Check sheet for the modelled part. Datum: model origin and axes. Units: mm. A direction names the side the tool comes from. Round coordinates to 2 decimals unless told otherwise and drop trailing zeros. Write each loop counter-clockwise with the first axis right and the second up, starting at its lowest first coordinate (ties: lowest second). Pieces come first, ordered by that corner, then holes. Notation, with made-up numbers: M -1,-26.75 L 19,-26.75 A19 cw 19,0.25 Z; hole C -36,21.5 d3. An arc over 180 degrees is marked long. Put each result on its own line as item: value.
```python
from build123d import *

# Parameters (mm, degrees)
SKETCH_1_W          = 48.3
SKETCH_1_H          = 28.3
EXTRUDE_1_DEPTH     = 1.6
SKETCH_3_W          = 25.5
SKETCH_3_H          = 17.8
EXTRUDE_2_DEPTH     = 0.7
SKETCH_4_W          = 17.4
SKETCH_4_H          = 15.8
EXTRUDE_3_DEPTH     = 2.3
SKETCH_5_W          = 6.4
SKETCH_5_H          = 7.4
EXTRUDE_4_DEPTH     = 2.4
CHAMFER_1_SIZE      = 0.5
SKETCH_6_R          = 0.6
CUT_EXTRUDE_1_DEPTH = 34.530359378


with BuildPart() as part:
    # 草图1 → 凸台-拉伸1 (new body)
    with BuildSketch(Plane(origin=(0, 0, 0), x_dir=(1, 0, 0), z_dir=(0, 1, 0))):
        Rectangle(SKETCH_1_W, SKETCH_1_H)
    extrude(amount=EXTRUDE_1_DEPTH)

    # 草图3 → 凸台-拉伸2 (add)
    with BuildSketch(Plane(origin=(0, 1.6, 0), x_dir=(1, 0, 0), z_dir=(0, 1, 0))):
        with Locations((-17.5, 0)):
            Rectangle(SKETCH_3_W, SKETCH_3_H)
    extrude(amount=EXTRUDE_2_DEPTH)

    # 草图4 → 凸台-拉伸3 (add)
    with BuildSketch(Plane(origin=(0, 2.3, 0), x_dir=(1, 0, 0), z_dir=(0, 1, 0))):
        with Locations((-14.45, 0)):
            Rectangle(SKETCH_4_W, SKETCH_4_H)
    extrude(amount=EXTRUDE_3_DEPTH)

    # 草图5 → 凸台-拉伸4 (add)
    with BuildSketch(Plane(origin=(0, 1.6, 0), x_dir=(1, 0, 0), z_dir=(0, 1, 0))):
        with Locations((21.65, 0)):
            Rectangle(SKETCH_5_W, SKETCH_5_H)
    extrude(amount=EXTRUDE_4_DEPTH)

    # 倒角1
    chamfer_1_edges = [part.edges().sort_by_distance(p)[0] for p in [
        (21.65, 4, -3.7),
        (21.65, 4, 3.7),
    ]]
    chamfer(chamfer_1_edges, length=CHAMFER_1_SIZE)

    # 草图6 → 切除-拉伸1 (cut, through all)
    with BuildSketch(Plane(origin=(0, 1.6, 0), x_dir=(1, 0, 0), z_dir=(0, 1, 0))):
        with Locations(Location((22.95, 12.7, 0), (0, 0, 270))):
            Circle(SKETCH_6_R)
        with Locations(Location((20.41, 12.7, 0), (0, 0, 270))):
            Circle(SKETCH_6_R)
        with Locations(Location((17.87, 12.7, 0), (0, 0, 270))):
            Circle(SKETCH_6_R)
        with Locations(Location((15.33, 12.7, 0), (0, 0, 270))):
            Circle(SKETCH_6_R)
        with Locations(Location((12.79, 12.7, 0), (0, 0, 270))):
            Circle(SKETCH_6_R)
        with Locations(Location((10.25, 12.7, 0), (0, 0, 270))):
            Circle(SKETCH_6_R)
        with Locations(Location((7.71, 12.7, 0), (0, 0, 270))):
            Circle(SKETCH_6_R)
        with Locations(Location((5.17, 12.7, 0), (0, 0, 270))):
            Circle(SKETCH_6_R)
        with Locations(Location((2.63, 12.7, 0), (0, 0, 270))):
            Circle(SKETCH_6_R)
        with Locations(Location((0.09, 12.7, 0), (0, 0, 270))):
            Circle(SKETCH_6_R)
        with Locations(Location((-2.45, 12.7, 0), (0, 0, 270))):
            Circle(SKETCH_6_R)
        with Locations(Location((-4.99, 12.7, 0), (0, 0, 270))):
            Circle(SKETCH_6_R)
        with Locations(Location((-7.53, 12.7, 0), (0, 0, 270))):
            Circle(SKETCH_6_R)
        with Locations(Location((-10.07, 12.7, 0), (0, 0, 270))):
            Circle(SKETCH_6_R)
        with Locations(Location((-12.61, 12.7, 0), (0, 0, 270))):
            Circle(SKETCH_6_R)
        with Locations(Location((-15.15, 12.7, 0), (0, 0, 270))):
            Circle(SKETCH_6_R)
        with Locations(Location((-17.69, 12.7, 0), (0, 0, 270))):
            Circle(SKETCH_6_R)
        with Locations(Location((-20.23, 12.7, 0), (0, 0, 270))):
            Circle(SKETCH_6_R)
        with Locations(Location((-22.77, 12.7, 0), (0, 0, 270))):
            Circle(SKETCH_6_R)
        with Locations(Location((20.41, -12.7, 0), (0, 0, 270))):
            Circle(SKETCH_6_R)
        with Locations(Location((17.87, -12.7, 0), (0, 0, 270))):
            Circle(SKETCH_6_R)
        with Locations(Location((15.33, -12.7, 0), (0, 0, 270))):
            Circle(SKETCH_6_R)
        with Locations(Location((12.79, -12.7, 0), (0, 0, 270))):
            Circle(SKETCH_6_R)
        with Locations(Location((10.25, -12.7, 0), (0, 0, 270))):
            Circle(SKETCH_6_R)
        with Locations(Location((7.71, -12.7, 0), (0, 0, 270))):
            Circle(SKETCH_6_R)
        with Locations(Location((5.17, -12.7, 0), (0, 0, 270))):
            Circle(SKETCH_6_R)
        with Locations(Location((2.63, -12.7, 0), (0, 0, 270))):
            Circle(SKETCH_6_R)
        with Locations(Location((0.09, -12.7, 0), (0, 0, 270))):
            Circle(SKETCH_6_R)
        with Locations(Location((-2.45, -12.7, 0), (0, 0, 270))):
            Circle(SKETCH_6_R)
        with Locations(Location((-4.99, -12.7, 0), (0, 0, 270))):
            Circle(SKETCH_6_R)
        with Locations(Location((-7.53, -12.7, 0), (0, 0, 270))):
            Circle(SKETCH_6_R)
        with Locations(Location((-10.07, -12.7, 0), (0, 0, 270))):
            Circle(SKETCH_6_R)
        with Locations(Location((-12.61, -12.7, 0), (0, 0, 270))):
            Circle(SKETCH_6_R)
        with Locations(Location((-15.15, -12.7, 0), (0, 0, 270))):
            Circle(SKETCH_6_R)
        with Locations(Location((-17.69, -12.7, 0), (0, 0, 270))):
            Circle(SKETCH_6_R)
        with Locations(Location((-20.23, -12.7, 0), (0, 0, 270))):
            Circle(SKETCH_6_R)
        with Locations(Location((-22.77, -12.7, 0), (0, 0, 270))):
            Circle(SKETCH_6_R)
        with Locations(Location((22.95, -12.7, 0), (0, 0, 270))):
            Circle(SKETCH_6_R)
    extrude(amount=-CUT_EXTRUDE_1_DEPTH, mode=Mode.SUBTRACT)


solid = part.part
```
1. Access from +Z, -Z, +X, -X, +Y, -Y to the whole of each face (thin tool, end or side, straight path). Record for faces 4 (the flat face through (24.15, 1, 0)), 5 (the cylindrical face through (-2.98, 0.81, -12.42)), 6 (the flat face through (-5.75, 3, 0)).
Computed values:
face 4: +Z, -Z, +X, -Y
face 5: +Y, -Y
face 6: +Z, -Z, +Y
2. Cross-section at B-B (z = 5). Enter the section's corners in (x, y), then the cut area to 3 significant figures.
Computed values:
outline: M -30.25,1.6 L -24.15,1.6 L -24.15,0 L 24.15,0 L 24.15,1.6 L -4.75,1.6 L -4.75,2.3 L -5.75,2.3 L -5.75,4.6 L -23.15,4.6 L -23.15,2.3 L -30.25,2.3 Z
area: 135 mm2
3. Release check for a two-part mould opening along Z. For faces 1 (the flat face through (-24.15, 1, 0)), 2 (the cylindrical face through (-7.35, 0.811, 13.272)), 3 (the flat face through (-15, 3, 7.9)) record: +Z half, -Z half, draft (parallel to the pull), parting line (faces both ways), or undercut.
Computed values:
face 1: draft
face 2: undercut
face 3: +Z half
4. Depth check by flat-ended pin: pin 1 Ø1.4 at (x, z) = (-4.99, 12.7) entering from +Y; pin 2 Ø0.7 at (x, y) = (-12, 3.5) entering from +Z; pin 3 Ø6.5 at (x, z) = (-28, 3.5) entering from -Y. Enter the tip coordinate at first touch or a pass-through.
Computed values:
pin 1: stops at y = 1.6
pin 2: stops at z = 7.9
pin 3: stops at y = 1.6
5. Scan lines: probe 1 along Z at (x, y) = (-15, 2.05); probe 2 along Y at (x, z) = (-23, 8.25); probe 3 along Y at (x, z) = (11, 3.25). Record each from-to range of solid material in increasing order.
Computed values:
probe 1: z = -8.9 to 8.9
probe 2: y = 0 to 2.3
probe 3: y = 0 to 1.6
6. Cross-section at A-A (x = 10.25). Enter the section's corners in (y, z).
Computed values:
outline: M 0,-14.15 L 1.6,-14.15 L 1.6,-13.3 L 0,-13.3 Z; M 0,-12.1 L 1.6,-12.1 L 1.6,12.1 L 0,12.1 Z; M 0,13.3 L 1.6,13.3 L 1.6,14.15 L 0,14.15 Z
7. Cross-section at C-C (x = 22.95). Enter the section's corners in (y, z).
Computed values:
outline: M 0,-14.15 L 1.6,-14.15 L 1.6,-13.3 L 0,-13.3 Z; M 0,-12.1 L 1.6,-12.1 L 1.6,-3.7 L 3.5,-3.7 L 4,-3.2 L 4,3.2 L 3.5,3.7 L 1.6,3.7 L 1.6,12.1 L 0,12.1 Z; M 0,13.3 L 1.6,13.3 L 1.6,14.15 L 0,14.15 Z
8. Cross-section at D-D (x = -14). Enter the section's corners in (y, z).
Computed values:
outline: M 0,-14.15 L 1.6,-14.15 L 1.6,-8.9 L 2.3,-8.9 L 2.3,-7.9 L 4.6,-7.9 L 4.6,7.9 L 2.3,7.9 L 2.3,8.9 L 1.6,8.9 L 1.6,14.15 L 0,14.15 Z
